```python
from build123d import *

# Parameters (mm, degrees)
F2_R = 0.8
F3_R = 0.2


with BuildPart() as f1:
    # F0 (on Front) → F1 (revolve)
    with BuildSketch(Plane.XZ):
        Polygon((-2.55, -2.47), (-2.55, 6.35), (-4.5, 6.35), (-4.5, 2.13), (-5, 2.13), (-5, 0), (-3.58, 0), (-3.58, -2.47), align=None)
    revolve(axis=Axis((0, 0, -0.888866), (0, 0, -1)))

    # F2
    f2_edges = [f1.edges().sort_by_distance(p)[0] for p in [
        (4.5, 0, 6.35),
    ]]
    fillet(f2_edges, radius=F2_R)

    # F3
    f3_edges = [f1.edges().sort_by_distance(p)[0] for p in [
        (2.55, 0, 6.35),
    ]]
    fillet(f3_edges, radius=F3_R)


solid = f1.part
```
Could you check a few things on this model? Use its own coordinates, in mm. A direction names the side the tool comes from. Coordinates: 2 decimals unless noted, no trailing zeros. Write each loop counter-clockwise with the first axis right and the second up, starting at its lowest first coordinate (ties: lowest second). Pieces come first, ordered by that corner, then holes. Notation, with made-up numbers: (-21.75, -24.5) - (-16.75, -24.5) arc R21 ccw to (-16.75, -18.5) - close; hole circle Ø2 at (24, 85.25). An arc over 180 degrees is marked (long way). Use a Markdown table: item, result.
Q1. Please list where these lines run through material, in increasing order: L1, parallel to Y at x = 0, z = 4; L2, parallel to Y at x = 0, z = -0.25; L3, parallel to Z at x = -4.5, y = 1.5.
Geometry check:
| item | result |
|---|---|
| L1 | y = -4.5 to -2.55, 2.55 to 4.5 |
| L2 | y = -3.58 to -2.55, 2.55 to 3.58 |
| L3 | z = 0 to 2.13 |
Q2. I'm going to push flat-ended pins straight in: pin 1 Ø5 at (y, z) = (-0.5, 5.5) entering from +X; pin 2 Ø1 at (x, y) = (-0.5, -1) entering from -Z; pin 3 Ø2 at (y, z) = (2.5, 0.5) entering from +X; pin 4 Ø1.5 at (x, z) = (-2, 1) entering from -Y. Where does each tip first touch, or does it pass through?
Geometry check:
| item | result |
|---|---|
| pin 1 | stops at x = 4.5 |
| pin 2 | passes through |
| pin 3 | stops at x = 4.77 |
| pin 4 | stops at y = -4.84 |
Q3. Which directions (+Z, -Z, +X, -X, +Y, -Y) give clear straight access to the entire face, cutting with the end or side of a thin tool? Please do faces 4 (the cylindrical face through (0.776, -3.495, -1.252)), 5 (the cylindrical face through (1.08, -4.88, 1.05)).
Geometry check:
| item | result |
|---|---|
| face 4 | -Z |
| face 5 | +Z, -Z |
Q4. Thinking about a two-plate mould opening in Y: for faces 1 (the cylindrical face through (-1.18, -2.26, 1.9)), 2 (the cylindrical face through (0.59, 4.46, 3.82)), 3 (the flat face through (0, 3, 6.35)), which applies, +Y half, -Y half, draft (parallel to the pull), parting line (faces both ways), or undercut?
Geometry check:
| item | result |
|---|---|
| face 1 | undercut |
| face 2 | parting line |
| face 3 | draft |
Q5. Imagine slicing it at A-A (x = 0). List the corners of the cut face in (y, z) for me, and give its area (3 significant figures).
Geometry check:
| item | result |
|---|---|
| outline | (-5, 0) - (-3.58, 0) - (-3.58, -2.47) - (-2.55, -2.47) - (-2.55, 6.15) arc R0.2 ccw to (-2.75, 6.35) - (-3.7, 6.35) arc R0.8 ccw to (-4.5, 5.55) - (-4.5, 2.13) - (-5, 2.13) - close; (2.55, -2.47) - (3.58, -2.47) - (3.58, 0) - (5, 0) - (5, 2.13) - (4.5, 2.13) - (4.5, 5.55) arc R0.8 ccw to (3.7, 6.35) - (2.75, 6.35) arc R0.2 ccw to (2.55, 6.15) - close |
| area | 31.7 mm2 |
